```python
from build123d import *

# Parameters (mm, degrees)
SKETCH_1_W          = 254.5
SKETCH_1_H          = 15
EXTRUDE_1_DEPTH     = 3
SKETCH_2_W          = 8
SKETCH_2_H          = 3
SKETCH_2_W_2        = 6
EXTRUDE_2_DEPTH     = 3
SKETCH_3_R          = 1
CUT_EXTRUDE_1_DEPTH = 3
FILLET_1_R          = 0.5
SKETCH_4_R          = 1.25
CUT_EXTRUDE_2_DEPTH = 10
FILLET_2_R          = 8


with BuildPart() as part:
    # 스케치1 → 보스-돌출1 (new body)
    with BuildSketch(Plane(origin=(0, 0, 0), x_dir=(0, 0, -1), z_dir=(1, 0, 0))):
        with Locations((127.25, 7.5)):
            Rectangle(SKETCH_1_W, SKETCH_1_H)
    extrude(amount=EXTRUDE_1_DEPTH)

    # 스케치2 → 보스-돌출2 (add)
    with BuildSketch(Plane(origin=(3, 0, 0), x_dir=(0, 0, -1), z_dir=(1, 0, 0))):
        with Locations((4, 16.5)):
            Rectangle(SKETCH_2_W, SKETCH_2_H)
        with Locations((251.5, 16.5)):
            Rectangle(SKETCH_2_W_2, SKETCH_2_H)
    extrude(amount=-EXTRUDE_2_DEPTH)

    # 스케치3 → 컷-돌출1 (cut)
    with BuildSketch(Plane(origin=(3, 0, 0), x_dir=(0, 0, -1), z_dir=(1, 0, 0))):
        with Locations((9, 15)):
            Circle(SKETCH_3_R)
        with Locations((247.5, 15)):
            Circle(SKETCH_3_R)
    extrude(amount=-CUT_EXTRUDE_1_DEPTH, mode=Mode.SUBTRACT)

    # 필렛1
    fillet_1_edges = [part.edges().sort_by_distance(p)[0] for p in [
        (1.5, 18, 0),
        (1.5, 18, -8),
        (1.5, 18, -254.5),
        (1.5, 18, -248.5),
    ]]
    fillet(fillet_1_edges, radius=FILLET_1_R)

    # 스케치4 → 컷-돌출2 (cut)
    with BuildSketch(Plane(origin=(3, 0, 0), x_dir=(0, 0, -1), z_dir=(1, 0, 0))):
        with Locations((225, 5)):
            Circle(SKETCH_4_R)
        with Locations((25, 5)):
            Circle(SKETCH_4_R)
    extrude(amount=-CUT_EXTRUDE_2_DEPTH, mode=Mode.SUBTRACT)

    # 필렛2
    fillet_2_edges = [part.edges().sort_by_distance(p)[0] for p in [
        (1.5, 0, -254.5),
    ]]
    fillet(fillet_2_edges, radius=FILLET_2_R)


solid = part.part
```
Can you work these out from the model? Positions are in its coordinate system, mm. Round coordinates to 2 decimals unless told otherwise and drop trailing zeros. Loops run counter-clockwise (first coordinate to the right, second up) from the corner with the lowest first, then second, coordinate; pieces in that order, holes last. Notation, with made-up numbers: (-25.5, 40.5) -> (0.5, 40.5) arc R23 cw to (0.5, 58.5) -> close; hole circle Ø6 at (-24, 8). An arc over 180 degrees is marked (long way). One line per item, written item: value. Start each with the question number.
1. If I drill on probe 1 along Y at (x, z) = (1.7, -25); probe 2 along Y at (x, z) = (2.2, -103.5); probe 3 along Z at (x, y) = (0.1, 2.5), over which ranges is the centre line in solid material (lowest first)?
2. For pin 1 (1 mm diameter, centred on x = 2.5, z = -172, fed in from +Y), with a flat end and sliding along its axis, tell me the tip position at first contact or that it passes through.
3. If we section it at A-A, the plane x = 2.2: Write out the boundary of the cut face in (y, z).
4. If we section it at B-B, the plane z = -165.5: Write out the boundary of the cut face in (x, y).
Calculated:
1. probe 1: y = 0 to 3.75, 6.25 to 15
1. probe 2: y = 0 to 15
1. probe 3: z = -252.31 to 0
2. pin 1: stops at y = 15
3. outline: (0, -246.5) arc R8 ccw to (8, -254.5) -> (17.5, -254.5) arc R0.5 ccw to (18, -254) -> (18, -249) arc R0.5 ccw to (17.5, -248.5) -> (15, -248.5) arc R1 cw to (15, -246.5) -> (15, -10) arc R1 cw to (15, -8) -> (17.5, -8) arc R0.5 ccw to (18, -7.5) -> (18, -0.5) arc R0.5 ccw to (17.5, 0) -> (0, 0) -> close; hole circle Ø2.5 at (5, -225); hole circle Ø2.5 at (5, -25)
4. outline: (0, 0) -> (3, 0) -> (3, 15) -> (0, 15) -> close
